Can you work these out from the model? Positions are in its coordinate system, mm. Face numbers are marked on the shaded views. A direction names the side the tool comes from. Coordinates: 2 decimals unless noted, no trailing zeros. Order: outer loops, then holes, each group sorted by start corner. A loop starts at its lowest first (then second) coordinate and runs counter-clockwise, first axis right, second up. Notation, with made-up numbers: (-12, 38) -> (32, 38) arc R21 ccw to (32, 44) -> close; hole circle Ø6 at (5, 81.5). An arc over 180 degrees is marked (long way). Answer as CSV lines item,"result".
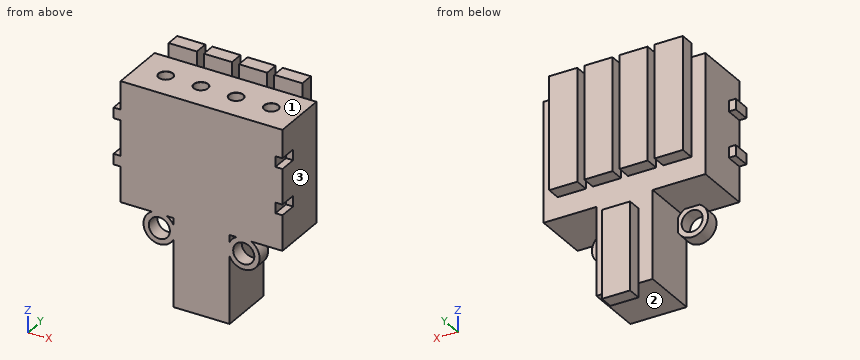
from build123d import *

# Parameters (mm, degrees)
SKETCH1_W                  = 8
SKETCH1_H                  = 17
CONNECTOR_BODY_DEPTH       = 8
SKETCH4_W                  = 4
SKETCH4_H                  = 16
CLAMP_DEPTH                = 2
CONNECTOR_PATTERN_COUNT    = 4
CONNECTOR_PATTERN_PITCH    = 5
SKETCH5_W                  = 8
SKETCH5_H                  = 12.5
SINGLE_BODY_DEPTH          = 8
SKETCH6_W                  = 1.5
SKETCH6_H                  = 2.500390225
CHAINING_NOBS_DEPTH        = 1
SKETCH7_W                  = 1
SKETCH7_H                  = 1.5
CHAINING_NOBS_CUTOUT_DEPTH = 2.50039
SKETCH8_W                  = 4
SKETCH8_H                  = 12.5
SINGLE_BODY_CLAMP_DEPTH    = 2
SKETCH9_R                  = 2.25
SKETCH9_R_2                = 1.5
MOUNTING_RINGS_DEPTH       = 2


with BuildPart() as part:
    # Sketch1 → connector_body (new body)
    with BuildSketch(Plane(origin=(0, 0, 0), x_dir=(1, 0, 0), z_dir=(0, 1, 0))):
        with Locations((4, 8.5)):
            Rectangle(SKETCH1_W, SKETCH1_H)
    connector_body = extrude(amount=CONNECTOR_BODY_DEPTH)

    # Sketch3 → cable_hole (revolve, cut)
    with BuildSketch(Plane(origin=(4, 4, 0), x_dir=(0, -1, 0), z_dir=(1, 0, 0))):
        Polygon((0, 0), (0, 10.600860619), (1, 10), (1, 0.025), (1.025, 0), align=None)
    cable_hole = revolve(axis=Axis((4, 4, 6.35), (0, 0, -1)), mode=Mode.SUBTRACT)

    # Sketch4 → clamp (add)
    with BuildSketch(Plane(origin=(0, 8, 0), x_dir=(1, 0, 0), z_dir=(0, 1, 0))):
        with Locations((4, 6)):
            Rectangle(SKETCH4_W, SKETCH4_H)
    clamp = extrude(amount=CLAMP_DEPTH)

    # connector_pattern: connector_body, cable_hole, clamp ×4
    with Locations(*[(i * CONNECTOR_PATTERN_PITCH, 0, 0) for i in range(1, CONNECTOR_PATTERN_COUNT)]):
        add(connector_body)
        add(cable_hole, mode=Mode.SUBTRACT)
        add(clamp)

    # Sketch5 → single_body (add)
    with BuildSketch(Plane(origin=(0, 8, 0), x_dir=(1, 0, 0), z_dir=(0, 1, 0))):
        with Locations((11.5, 23.25)):
            Rectangle(SKETCH5_W, SKETCH5_H)
    extrude(amount=-SINGLE_BODY_DEPTH)

    # Sketch6 → chaining_nobs (add)
    with BuildSketch(Plane.ZY):
        with Locations((-11.25, 1.250195113)):
            Rectangle(SKETCH6_W, SKETCH6_H)
        with Locations((-4.75, 1.250195113)):
            Rectangle(SKETCH6_W, SKETCH6_H)
    extrude(amount=CHAINING_NOBS_DEPTH)

    # Sketch7 → chaining_nobs_cutout (cut)
    with BuildSketch(Plane.XZ):
        with Locations((22.5, -4.75)):
            Rectangle(SKETCH7_W, SKETCH7_H)
        with Locations((22.5, -11.25)):
            Rectangle(SKETCH7_W, SKETCH7_H)
    extrude(amount=-CHAINING_NOBS_CUTOUT_DEPTH, mode=Mode.SUBTRACT)

    # Sketch8 → single_body_clamp (add)
    with BuildSketch(Plane(origin=(0, 8, 0), x_dir=(1, 0, 0), z_dir=(0, 1, 0))):
        with Locations((11.5, 25.25)):
            Rectangle(SKETCH8_W, SKETCH8_H)
    extrude(amount=SINGLE_BODY_CLAMP_DEPTH)

    # Sketch9 → mounting_rings (add)
    # profile 1 of 2: a face of its own
    with BuildSketch(Plane.XZ):
        with Locations((5.5, -19)):
            Circle(SKETCH9_R)
        with Locations(Location((5.5, -19, 0), (0, 0, 270))):
            Circle(SKETCH9_R_2, mode=Mode.SUBTRACT)
    # profile 2 of 2: a face of its own
    with BuildSketch(Plane.XZ):
        with Locations((17.5, -19)):
            Circle(SKETCH9_R)
        with Locations(Location((17.5, -19, 0), (0, 0, 270))):
            Circle(SKETCH9_R_2, mode=Mode.SUBTRACT)
    extrude(amount=-MOUNTING_RINGS_DEPTH)


solid = part.part
Q1. Imagine slicing it at A-A (x = 5.5). List the corners of the cut face in (y, z) for me, and give its area (4 significant figures).
Solution:
outline,"(0, -21.25) -> (2, -21.25) -> (2, -20.5) -> (0, -20.5) -> close; (0, -17.5) -> (2, -17.5) -> (2, -17) -> (8, -17) -> (8, -14) -> (10, -14) -> (10, 2) -> (8, 2) -> (8, 0) -> (0, 0) -> close"
area,"170.5 mm2"
Q2. If I drill on line 1 (X direction, y = 8.25, z = -8); line 2 (X direction, y = 4, z = -2.5); line 3 (X direction, y = 0.8, z = -19), over which ranges is the centre line in solid material (lowest first)?
Solution:
line 1,"2 to 6, 7 to 11, 12 to 16, 17 to 21"
line 2,"0 to 3, 5 to 8, 10 to 13, 15 to 18, 20 to 23"
line 3,"3.25 to 4, 7 to 16, 19 to 19.75"
Q3. Imagine slicing it at B-B (z = -3.5). List the corners of the cut face in (x, y) for me.
Solution:
outline,"(0, 0) -> (23, 0) -> (23, 8) -> (21, 8) -> (21, 10) -> (17, 10) -> (17, 8) -> (16, 8) -> (16, 10) -> (12, 10) -> (12, 8) -> (11, 8) -> (11, 10) -> (7, 10) -> (7, 8) -> (6, 8) -> (6, 10) -> (2, 10) -> (2, 8) -> (0, 8) -> close; hole circle Ø2 at (4, 4); hole circle Ø2 at (9, 4); hole circle Ø2 at (14, 4); hole circle Ø2 at (19, 4)"
Q4. Imagine slicing it at D-D (x = 10.5). List the corners of the cut face in (y, z) for me.
Solution:
outline,"(0, -29.5) -> (8, -29.5) -> (8, -31.5) -> (10, -31.5) -> (10, -19) -> (8, -19) -> (8, -14) -> (10, -14) -> (10, 2) -> (8, 2) -> (8, 0) -> (0, 0) -> close"
Q5. For P1, Ø1.8, axis at x = 19, y = 4, coming from the +Z side; P2, Ø1.1, axis at x = -0.5, z = -11, coming from the +Y side; P3, Ø1, axis at y = 1.5, z = -22.5, coming from the -X side, each with a flat end and sliding along its axis, tell me the tip position at first contact or that it passes through.
Solution:
P1,"z = -10.06"
P2,"y = 8"
P3,"x = 7.5"
Q6. Which directions (+Z, -Z, +X, -X, +Y, -Y) give clear straight access to the entire face, cutting with the end or side of a thin tool? Please do the marked faces 1, 2 and 3.
Solution:
face 1,"+Z, +X, -X, -Y"
face 2,"-Z, +X, -X, -Y"
face 3,"+Z, -Z, +X, +Y, -Y"
Q7. Imagine slicing it at C-C (y = 6.75). List the corners of the cut face in (x, z) for me.
Solution:
outline,"(0, -17) -> (7.5, -17) -> (7.5, -29.5) -> (15.5, -29.5) -> (15.5, -17) -> (23, -17) -> (23, 0) -> (0, 0) -> close"
